from build123d import *

# Parameters (mm, degrees)
F1_DEPTH = 3
F2_R     = 1.25
F2_R_2   = 2.5
F2_R_3   = 1
F2_R_4   = 10
F2_R_5   = 1.5
F3_DEPTH = 3.001
F4_R     = 5


with BuildPart() as f1:
    # F0 (on Top) → F1 (new body)
    with BuildSketch(Plane.XY):
        with BuildLine():
            ThreePointArc((8.466655, -22.315393), (22.987813, -30.509533), (31.665328, -44.747113))
            ThreePointArc((31.665328, -44.747113), (49.143921, -49.143921), (44.747113, -31.665328))
            ThreePointArc((44.747113, -31.665328), (21.213203, 0), (44.747113, 31.665328))
            ThreePointArc((44.747113, 31.665328), (49.143921, 49.143921), (31.665328, 44.747113))
            ThreePointArc((31.665328, 44.747113), (0, 21.213203), (-31.665328, 44.747113))
            ThreePointArc((-31.665328, 44.747113), (-49.143921, 49.143921), (-44.747113, 31.665328))
            ThreePointArc((-44.747113, 31.665328), (-21.213203, 0), (-44.747113, -31.665328))
            ThreePointArc((-44.747113, -31.665328), (-49.143921, -49.143921), (-31.665328, -44.747113))
            ThreePointArc((-31.665328, -44.747113), (-22.780732, -30.311029), (-7.910816, -22.173328))
            Line((-7.910816, -22.173328), (-5.631352, -28.306246))
            ThreePointArc((-5.631352, -28.306246), (-0.249426, -32.215765), (5.438293, -28.766226))
            Line((5.438293, -28.766226), (8.466655, -22.315393))
        make_face()
    extrude(amount=F1_DEPTH)

    # F2 (on face) → F3 (cut, through all)
    with BuildSketch(Plane.XY.offset(3)):
        with Locations((0, -14.142136)):
            Circle(F2_R)
        with Locations((-14.142136, 0)):
            Circle(F2_R)
        with Locations((0, 14.142136)):
            Circle(F2_R)
        with Locations((14.142136, 0)):
            Circle(F2_R)
        with Locations((-41.7193, -41.7193)):
            Circle(F2_R_2)
        with Locations((41.7193, -41.7193)):
            Circle(F2_R_2)
        with Locations((41.7193, 41.7193)):
            Circle(F2_R_2)
        with Locations((-41.7193, 41.7193)):
            Circle(F2_R_2)
        with Locations((-35.7193, 41.7193)):
            Circle(F2_R_3)
        with Locations((-41.7193, 35.7193)):
            Circle(F2_R_3)
        with Locations((-47.7193, 41.7193)):
            Circle(F2_R_3)
        with Locations((-41.7193, 47.7193)):
            Circle(F2_R_3)
        with Locations((35.7193, 41.7193)):
            Circle(F2_R_3)
        with Locations((47.7193, 41.7193)):
            Circle(F2_R_3)
        with Locations((41.7193, 47.7193)):
            Circle(F2_R_3)
        with Locations((41.7193, 35.7193)):
            Circle(F2_R_3)
        with Locations((41.7193, -35.7193)):
            Circle(F2_R_3)
        with Locations((35.7193, -41.7193)):
            Circle(F2_R_3)
        with Locations((41.7193, -47.7193)):
            Circle(F2_R_3)
        with Locations((47.7193, -41.7193)):
            Circle(F2_R_3)
        with Locations((-47.7193, -41.7193)):
            Circle(F2_R_3)
        with Locations((-41.7193, -47.7193)):
            Circle(F2_R_3)
        with Locations((-35.7193, -41.7193)):
            Circle(F2_R_3)
        with Locations((-41.7193, -35.7193)):
            Circle(F2_R_3)
        Circle(F2_R_4)
        with Locations((-12, 12)):
            Circle(F2_R_5)
        with Locations((12, 12)):
            Circle(F2_R_5)
        with Locations((0, -26)):
            Circle(F2_R_5)
    extrude(amount=-F3_DEPTH, mode=Mode.SUBTRACT)

    # F4
    f4_edges = [f1.edges().sort_by_distance(p)[0] for p in [
        (-7.910816, -22.173328, 1.5),
        (8.466655, -22.315393, 1.5),
    ]]
    fillet(f4_edges, radius=F4_R)


solid = f1.part
Read the model definition and answer for the solid it produces. Units are mm, in the model's axes. A direction names the side the tool comes from. Give positions to 0.01 mm unless a question says otherwise; leave off trailing zeros. Loops run counter-clockwise (first coordinate to the right, second up) from the corner with the lowest first, then second, coordinate; pieces in that order, holes last. Notation, with made-up numbers: (-18, -38.75) -> (7, -38.75) arc R14 ccw to (7, -26.75) -> close; hole circle Ø3 at (-27.5, -4.75). An arc over 180 degrees is marked (long way). Answer as CSV lines item,"result".
Item 1: Find section B-B on y = 0. Give the vertices of the cut face in (x, z).
Returned:
outline,"(-21.21, 0) -> (-15.39, 0) -> (-15.39, 3) -> (-21.21, 3) -> close; (-12.89, 0) -> (-10, 0) -> (-10, 3) -> (-12.89, 3) -> close; (10, 0) -> (12.89, 0) -> (12.89, 3) -> (10, 3) -> close; (15.39, 0) -> (21.21, 0) -> (21.21, 3) -> (15.39, 3) -> close"
Item 2: Find section D-D on z = 0.65. State how many separate pieces and enclosed holes the cut face has, plus the area to 3 significant figures.
Returned:
separate pieces,"1"
enclosed holes,"28"
area,"4,030 mm²"
Item 3: For faces 4 (the face through (-43.56, 43.41, 1.52)), 5 (the face through (5.99, -27.59, 1.48)), determine the directions among +Z, -Z, +X, -X, +Y, -Y from which every point of the face is accessible in a straight line to the end or side of a thin tool.
Returned:
face 4,"+Z, -Z"
face 5,"+Z, -Z, -Y"
Item 4: Determine the mould class of faces 1 (the face through (-48.926, 49.355, 1.479)), 2 (the face through (-1, -11, 3)), 3 (the face through (-0.35, -32.21, 1.48)) for opening direction Y: +Y half, -Y half, draft (parallel to the pull), parting line (faces both ways), or undercut.
Returned:
face 1,"undercut"
face 2,"draft"
face 3,"-Y half"
Item 5: Find section C-C on y = 33.5. Give the vertices of the cut face in (x, z).
Returned:
outline,"(-48.25, 0) -> (-25.72, 0) -> (-25.72, 3) -> (-48.25, 3) -> close; (25.72, 0) -> (48.25, 0) -> (48.25, 3) -> (25.72, 3) -> close"
Item 6: Each of these flat-tipped pins is pushed along its axis until it touches: pin 1 (1 mm diameter, centred on y = 16.5, z = 0.5, fed in from +X); pin 2 (6 mm diameter, centred on x = 41.72, y = -41.72, fed in from -Z); pin 3 (1.2 mm diameter, centred on x = 41.72, y = 47.72, fed in from -Z); pin 4 (1 mm diameter, centred on x = 8.5, z = 1.5, fed in from -Y). Where does it stop, or does it pass through?
Returned:
pin 1,"stops at x = 25.92"
pin 2,"stops at z = 0"
pin 3,"passes through"
pin 4,"stops at y = -24.56"
Item 7: Find section A-A on x = 0. Give the vertices of the cut face in (y, z), plus the area to 3 significant figures.
Returned:
outline,"(-32.22, 0) -> (-27.5, 0) -> (-27.5, 3) -> (-32.22, 3) -> close; (-24.5, 0) -> (-15.39, 0) -> (-15.39, 3) -> (-24.5, 3) -> close; (-12.89, 0) -> (-10, 0) -> (-10, 3) -> (-12.89, 3) -> close; (10, 0) -> (12.89, 0) -> (12.89, 3) -> (10, 3) -> close; (15.39, 0) -> (21.21, 0) -> (21.21, 3) -> (15.39, 3) -> close"
area,"76.3 mm²"
Item 8: Consider line 1 (Y direction, x = 44, z = 0.55); line 2 (X direction, y = -28.5, z = 0.45); line 3 (X direction, y = 47.5, z = 0.85). Determine where each line is inside the solid, lowest interval first. Write a range as [from, to].
Returned:
line 1,"y = [-51.97, -42.74], [-40.7, -31.43], [31.43, 40.7], [42.74, 51.97]"
line 2,"x = [-37.51, -20.71], [-5.56, 5.56], [20.71, 37.51]"
line 3,"x = [-50.48, -42.69], [-40.74, -32.95], [32.95, 40.74], [42.69, 50.48]"
